Autodesk Inventor part; units mm, degrees
ref_plane "YZ Plane" through (0, 0, 0) normal (1, 0, 0) x (0, 1, 0)
ref_plane "XZ Plane" through (0, 0, 0) normal (0, 1, 0) x (-1, 0, 0)
ref_plane "XY Plane" through (0, 0, 0) normal (0, 0, 1) x (1, 0, 0)
sketch "Sketch1" plane through (0, 0, 0) normal (0, 0, 1) x (1, 0, 0)
  line L0 (-6.25, -5.7997) -> (6.25, -5.7997)
  arc A0 (6.25, -5.7997) -> (6.25, 5.7997) centre (6.25, 0) ccw
  line L1 (6.25, 5.7997) -> (-6.25, 5.7997)
  arc A1 (-6.25, 5.7997) -> (-6.25, -5.7997) centre (-6.25, 0) ccw
  point P0 (0, 0)
  point P1 (0, 0)
extrude "Extrusion1" add sketch "Sketch1" against normal blind 0.9906
sketch "Sketch2" plane through (0, 0, 0) normal (0, 0, 1) x (1, 0, 0)
  line L0 (-6.25, 6.2997) -> (-4.25, 6.2997)
  line L1 (-6.25, 5.7997) -> (-6.25, 6.2997)
  line L2 (-4.25, 5.7997) -> (-6.25, 5.7997)
  line L3 (-4.25, 6.2997) -> (-4.25, 5.7997)
  line L4 (-6.25, 4.2997) -> (-6.25, 5.7997)
  line L5 (-4.25, 5.7997) -> (-4.25, 4.2997)
  line L6 (-4.25, 4.2997) -> (-6.25, 4.2997)
  line L7 (4.25, 6.2997) -> (6.25, 6.2997)
  line L8 (4.25, 5.7997) -> (4.25, 6.2997)
  line L9 (6.25, 6.2997) -> (6.25, 5.7997)
  line L10 (4.25, 4.2997) -> (4.25, 5.7997)
  line L11 (6.25, 5.7997) -> (6.25, 4.2997)
  line L12 (6.25, 4.2997) -> (4.25, 4.2997)
  line L13 (-4.25, -6.2997) -> (-6.25, -6.2997)
  line L14 (-4.25, -5.7997) -> (-4.25, -6.2997)
  line L15 (-6.25, -5.7997) -> (-4.25, -5.7997)
  line L16 (-6.25, -6.2997) -> (-6.25, -5.7997)
  line L17 (-6.25, -5.7997) -> (-6.25, -4.2997)
  line L18 (-6.25, -4.2997) -> (-4.25, -4.2997)
  line L19 (-4.25, -4.2997) -> (-4.25, -5.7997)
  line L20 (6.25, -5.2997) -> (6.25, -6.2997)
  line L21 (4.25, -6.2997) -> (4.25, -5.7997)
  line L22 (6.25, -6.2997) -> (4.25, -6.2997)
  line L23 (4.25, -5.7997) -> (4.25, -4.2997)
  line L24 (4.25, -4.2997) -> (6.25, -4.2997)
  line L25 (6.25, -4.2997) -> (6.25, -5.7997)
  point P0 (0, 0)
  point P1 (6.25, 0)
  point P2 (-6.25, 0)
  point P3 (0, 0)
extrude "Extrusion2" add sketch "Sketch2" along normal blind 0.9906
chamfer "Chamfer1" distance 0.508 distance2 0.9906 1 edges at (-5.25, 6.2997, 0.9906) measured on face at (-4.9167, 6.2997, 0.3302)
chamfer "Chamfer2" distance 0.508 distance2 0.9906 1 edges at (5.25, 6.2997, 0.9906) measured on face at (5.5833, 6.2997, 0.3302)
chamfer "Chamfer3" distance 0.508 distance2 0.9906 1 edges at (5.25, -6.2997, 0.9906) measured on face at (4.9167, -6.2997, 0.3302)
chamfer "Chamfer4" distance 0.508 distance2 0.9906 1 edges at (-5.25, -6.2997, 0.9906) measured on face at (-5.5833, -6.2997, 0.3302)
properties part number "276-2243" material "ABS Plastic"
Work out the finished part from the listing and answer in its coordinate system (mm). A direction names the side the tool comes from. Round coordinates to 2 decimals unless told otherwise and drop trailing zeros. Loops run counter-clockwise (first coordinate to the right, second up) from the corner with the lowest first, then second, coordinate; pieces in that order, holes last. Notation, with made-up numbers: M -13.75,-39.5 L -5.75,-39.5 A21 cw -5.75,-31.5 Z; hole C -27.75,67 d7. An arc over 180 degrees is marked long. One line per question, with ' | ' between items.
Q1. Find section B-B, the plane y = 0. Give the vertices of the cut face in (x, z).
Conclusion:
outline: M -12.05,-0.99 L 12.05,-0.99 L 12.05,0 L -12.05,0 Z
Q2. Each of these flat-tipped pins is pushed along its axis until it touches: pin 1 Ø1 at (y, z) = (2, 0) entering from +X; pin 2 Ø0.5 at (y, z) = (5, 0.5) entering from -X; pin 3 Ø1.1 at (x, z) = (-2.5, -0.5) entering from +Y. Where does it stop, or does it pass through?
Conclusion:
pin 1: stops at x = 11.85 | pin 2: stops at x = -6.25 | pin 3: stops at y = 5.8
Q3. The mould has two halves that part along X. Classify faces 1 (the flat face through (4.25, -5.3, 0.5)), 2 (the flat face through (5.2, -4.3, 0.5)), 3 (the flat face through (-6.25, -5.3, 0.5)): +X half, -X half, draft (parallel to the pull), parting line (faces both ways), or undercut.
Conclusion:
face 1: undercut | face 2: draft | face 3: -X half
Q4. Find section A-A, the plane x = 4.5. Give the vertices of the cut face in (y, z), then the cut area to 3 significant figures.
Conclusion:
outline: M -6.3,0 L -5.8,0 L -5.8,-0.99 L 5.8,-0.99 L 5.8,0 L 6.3,0 L 6.3,0.48 L 5.31,0.99 L 4.3,0.99 L 4.3,0 L -4.3,0 L -4.3,0.99 L -5.31,0.99 L -6.3,0.48 Z | area: 14.9 mm2
Q5. A tool of negligible diameter and unlimited length cuts with its end or side. For faces 4 (the flat face through (5.3, 4.3, 0.5)), 5 (the flat face through (6.25, 5.3, 0.5)), 6 (the flat face through (0.1, 5.8, -0.5)), 7 (the flat face through (-6.25, 5.3, 0.5)), from which of +Z, -Z, +X, -X, +Y, -Y can it reach the whole face along a straight path? Write none if from no direction.
Conclusion:
face 4: +Z, +X, -X | face 5: +Z, +X, +Y, -Y | face 6: -Z, +X, -X, +Y | face 7: +Z, -X, +Y, -Y
Q6. Consider line 1 along Y through (x, z) = (-3, -0.75); line 2 along Z through (x, y) = (1.25, 0); line 3 along X through (y, z) = (0.25, -0.8). Determine where each line is inside the solid, lowest interval first. Write a range as from..to.
Conclusion:
line 1: y = -5.8..5.8 | line 2: z = -0.99..0 | line 3: x = -12.04..12.04
Q7. Find section C-C, the plane x = -1. Give the vertices of the cut face in (y, z), then the cut area to 3 significant figures.
Conclusion:
outline: M -5.8,-0.99 L 5.8,-0.99 L 5.8,0 L -5.8,0 Z | area: 11.5 mm2
